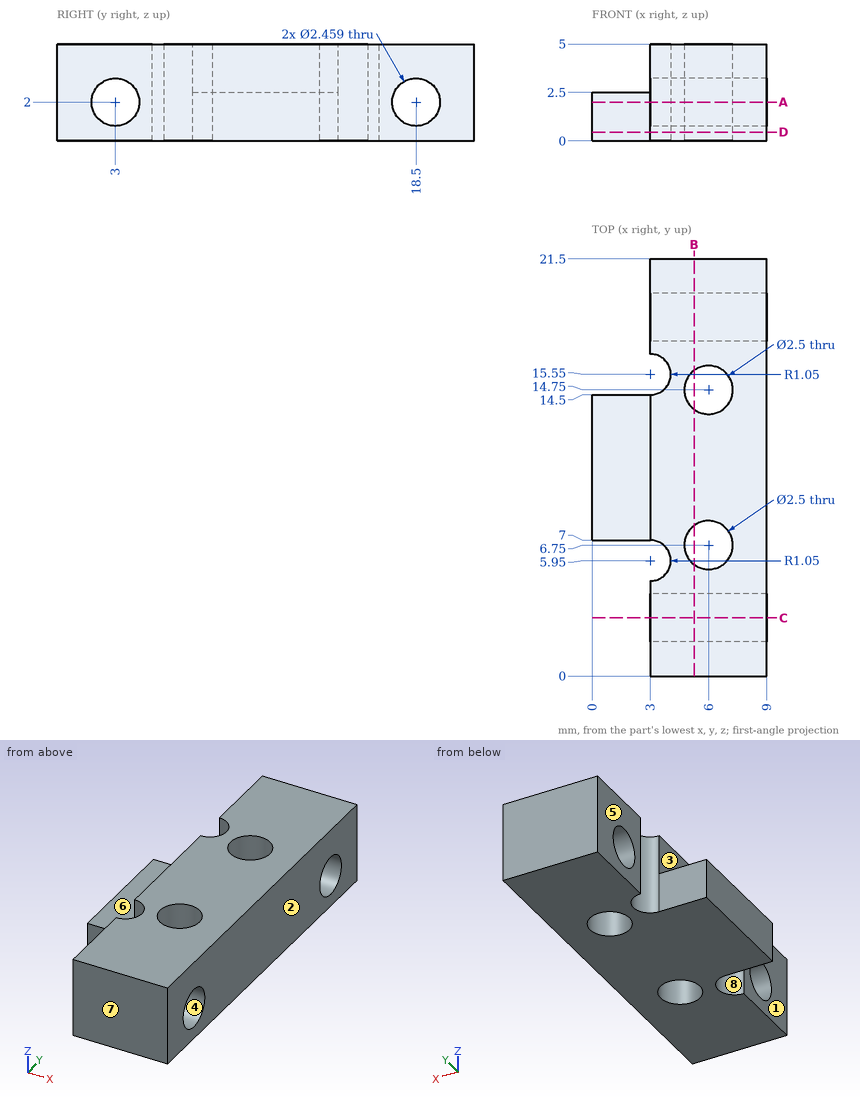
Print and shaded views of the part. All mm, measured from the part's lowest x, y and z. A direction names the side the tool comes from. Give positions to 0.01 mm unless a question says otherwise; leave off trailing zeros. Write each loop counter-clockwise with the first axis right and the second up, starting at its lowest first coordinate (ties: lowest second). Pieces come first, ordered by that corner, then holes. Notation, with made-up numbers: (46, 76.5) -> (97, 76.5) arc R13 cw to (97, 94.5) -> close; hole circle Ø10 at (-32.5, -14). An arc over 180 degrees is marked (long way). Write each question's results on one line, items separated by ' | '.
1. Cut at B-B, the plane x = 5.25. Write the cut outline in (y, z).
Geometry check:
outline: (0, 0) -> (5.75, 0) -> (5.75, 5) -> (0, 5) -> close; (7.75, 0) -> (13.75, 0) -> (13.75, 5) -> (7.75, 5) -> close; (15.75, 0) -> (21.5, 0) -> (21.5, 5) -> (15.75, 5) -> close; hole circle Ø2.46 at (3, 2); hole circle Ø2.46 at (18.5, 2)
2. Wall check: probe 1 along Y at (x, z) = (6, 4.7); probe 2 along Y at (x, z) = (6, 3.1); probe 3 along X at (y, z) = (14, 4). Give the ranges that are in metal, low to high. Write a range as [from, to].
Geometry check:
probe 1: [0, 5.5], [8, 13.5], [16, 21.5] | probe 2: [0, 2.45], [3.55, 5.5], [8, 13.5], [16, 17.95], [19.05, 21.5] | probe 3: [3, 5], [7, 9]
3. Cut at A-A, the plane z = 2. Write the cut outline in (x, y), then the cut area to 3 significant figures.
Geometry check:
outline: (0, 7) -> (3, 7) arc R1.05 cw to (3, 4.9) -> (3, 4.23) -> (9, 4.23) -> (9, 17.27) -> (3, 17.27) -> (3, 16.6) arc R1.05 cw to (3, 14.5) -> (0, 14.5) -> close; (3, 0) -> (9, 0) -> (9, 1.77) -> (3, 1.77) -> close; (3, 19.73) -> (9, 19.73) -> (9, 21.5) -> (3, 21.5) -> close; hole circle Ø2.5 at (6, 6.75); hole circle Ø2.5 at (6, 14.75) | area: 109 mm²
4. Two-plate mould, pull along Y, no slides. Class the marked faces 6, 7 and 8: pulls with the +Y half, pulls with the -Y half, needs draft (parallel to the pull), parting line crosses it, or undercut.
Geometry check:
face 6: needs draft | face 7: pulls with the -Y half | face 8: undercut
5. Drop flat-ended pins along their axis: P1, Ø1.2, axis at x = 2, z = 1.5, coming from the +Y side; P2, Ø3, axis at x = 6, y = 6.75, coming from the -Z side; P3, Ø2.5, axis at x = 1, y = 11, coming from the +Z side; P4, Ø2, axis at y = 9, z = 4.5, coming from the -X side. Give the stop position or say it passes through.
Geometry check:
P1: y = 14.5 | P2: z = 0 | P3: z = 2.5 | P4: x = 3
6. Which spindle directions (+Z, -Z, +X, -X, +Y, -Y) get a long thin tool onto all of the face, cutting with end or side? Do the marked faces 1, 2, 3, 4 and 5. Say none if no direction does.
Geometry check:
face 1: +Z, -Z, -X, -Y | face 2: +Z, -Z, +X, +Y, -Y | face 3: +Z, -X, +Y, -Y | face 4: +X, -X | face 5: +Z, -Z, -X, +Y
7. Cut at C-C, the plane y = 3. Write the cut outline in (x, z).
Geometry check:
outline: (3, 0) -> (9, 0) -> (9, 0.77) -> (3, 0.77) -> close; (3, 3.23) -> (9, 3.23) -> (9, 5) -> (3, 5) -> close
8. Cut at D-D, the plane z = 0.45. Write the cut outline in (x, y), then the cut area to 3 significant figures.
Geometry check:
outline: (0, 7) -> (3, 7) arc R1.05 cw to (3, 4.9) -> (3, 0) -> (9, 0) -> (9, 21.5) -> (3, 21.5) -> (3, 16.6) arc R1.05 cw to (3, 14.5) -> (0, 14.5) -> close; hole circle Ø2.5 at (6, 6.75); hole circle Ø2.5 at (6, 14.75) | area: 138 mm²
